Study the drawing (mm; zero at the part's minimum x, y, z) and answer. A direction names the side the tool comes from. Give positions to 0.01 mm unless a question says otherwise; leave off trailing zeros. Write each loop counter-clockwise with the first axis right and the second up, starting at its lowest first coordinate (ties: lowest second). Pieces come first, ordered by that corner, then holes. Notation, with made-up numbers: (16.5, 33) -> (37.5, 33) arc R28 ccw to (37.5, 51) -> close; hole circle Ø3 at (40.25, 61). An arc over 180 degrees is marked (long way). Put each result on its own line as item: value. Start each with the question number.
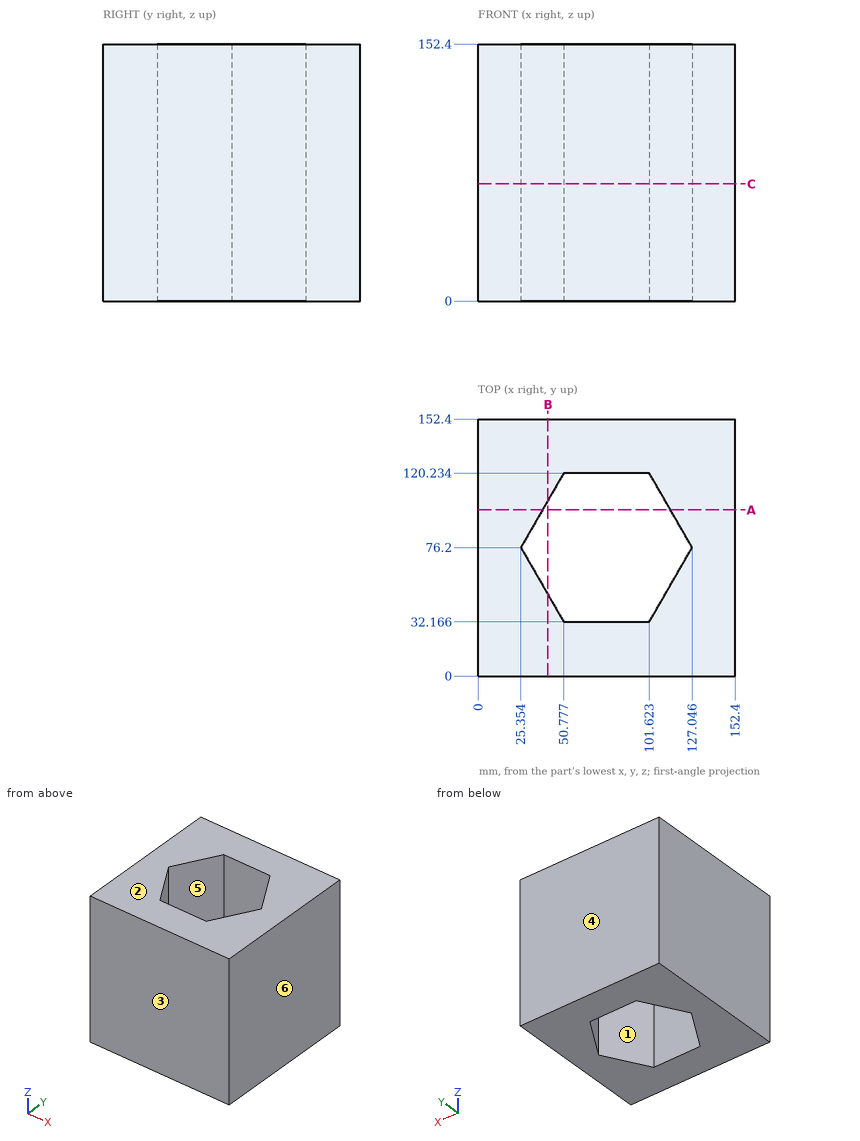
1) For a pull along Y with two mould halves and no side action, classify the marked faces 3, 4, 5 and 6 as pulls with the +Y half, pulls with the -Y half, needs draft (parallel to the pull), parting line crosses it, or undercut.
2) For the marked faces 1 and 2, determine the directions among +Z, -Z, +X, -X, +Y, -Y from which every point of the face is accessible in a straight line to the end or side of a thin tool.
3) A cutting plane is placed at B-B on x = 41.5. Give the vertices of the cut face in (y, z) (1 decimal).
4) A cutting plane is placed at C-C on z = 69.5. Give the vertices of the cut face in (x, y).
5) A cutting plane is placed at A-A on y = 98.5. Give the vertices of the cut face in (x, z), and give its area (3 significant figures).
6) Straight lines are drawn through the part: line 1 (Y direction, x = 78.5, z = 61.5); line 2 (X direction, y = 32.5, z = 66.5) (1 decimal); line 3 (Y direction, x = 123, z = 143) (1 decimal). For each, find the intervals that lie inside material, in ascending order. Write a range as [from, to].
Results found:
1. face 3: pulls with the -Y half
1. face 4: pulls with the +Y half
1. face 5: undercut
1. face 6: needs draft
2. face 1: +Z, -Z
2. face 2: +Z, +X, -X, +Y, -Y
3. outline: (0, 0) -> (48.2, 0) -> (48.2, 152.4) -> (0, 152.4) -> close; (104.2, 0) -> (152.4, 0) -> (152.4, 152.4) -> (104.2, 152.4) -> close
4. outline: (0, 0) -> (152.4, 0) -> (152.4, 152.4) -> (0, 152.4) -> close; hole (25.35, 76.2) -> (50.78, 32.17) -> (101.62, 32.17) -> (127.05, 76.2) -> (101.62, 120.23) -> (50.78, 120.23) -> close
5. outline: (0, 0) -> (38.23, 0) -> (38.23, 152.4) -> (0, 152.4) -> close; (114.17, 0) -> (152.4, 0) -> (152.4, 152.4) -> (114.17, 152.4) -> close
5. area: 11,700 mm²
6. line 1: y = [0, 32.17], [120.23, 152.4]
6. line 2: x = [0, 50.6], [101.8, 152.4]
6. line 3: y = [0, 69.2], [83.2, 152.4]
